Could you check a few things on this model? Use its own coordinates, in mm. Face numbers are marked on the shaded views. A direction names the side the tool comes from. Round coordinates to 2 decimals unless told otherwise and drop trailing zeros. Loops run counter-clockwise (first coordinate to the right, second up) from the corner with the lowest first, then second, coordinate; pieces in that order, holes last. Notation, with made-up numbers: (-21.75, -31.5) -> (31.25, -31.5) arc R10 cw to (31.25, -25.5) -> close; hole circle Ø11 at (-6.5, 23). An arc over 180 degrees is marked (long way). Write each question's results on one line, items separated by ' | '. Start each with the question number.
1) For P1, Ø4, axis at x = -231.5, y = 231.5, coming from the +Z side; P2, Ø8, axis at x = 100.5, z = -116.5, coming from the +Y side; P3, Ø5, axis at x = 156, y = 289.5, coming from the +Z side, each with a flat end and sliding along its axis, tell me the tip position at first contact or that it passes through.
2) Imagine slicing it at A-A, the plane y = 55.5. List the corners of the cut face in (x, z) for me.
3) We'd pull the mould along Z, two halves only. Please class the marked faces 1, 2 and 3: pulls with the +Z half, pulls with the -Z half, needs draft (parallel to the pull), parting line crosses it, or undercut.
4) Which directions (+Z, -Z, +X, -X, +Y, -Y) give clear straight access to the entire face, cutting with the end or side of a thin tool? Please do the marked faces 4 and 5.
5) Imagine slicing it at C-C, the plane z = -59.5. List the corners of the cut face in (x, y) for me.
6) If I drill on probe 1 along Z at (x, y) = (328, 100); probe 2 along Y at (x, z) = (423, 38); probe 3 along Z at (x, y) = (368, 274), over which ranges is the centre line in solid material (lowest first)?
7) Imagine slicing it at B-B, the plane x = -215.5. List the corners of the cut face in (y, z) for me, plus the area to 3 significant figures.
8) Imagine slicing it at D-D, the plane y = 220. List the corners of the cut face in (x, z) for me, plus the area to 3 significant figures.
Autodesk Inventor part; units mm, degrees
ref_plane "YZ Plane" through (0, 0, 0) normal (1, 0, 0) x (0, 1, 0)
ref_plane "XZ Plane" through (0, 0, 0) normal (0, 1, 0) x (-1, 0, 0)
ref_plane "XY Plane" through (0, 0, 0) normal (0, 0, 1) x (1, 0, 0)
sketch "Sketch1" plane through (0, 0, 0) normal (0, 1, 0) x (-1, 0, 0)
  line L0 (500, 200) -> (-500, 200)
  line L1 (-500, 200) -> (-500, -200)
  line L2 (-500, -200) -> (500, -200)
  line L3 (500, -200) -> (500, 200)
  line L4 (500, 200) -> (-500, -200) construction
  line L5 (-500, 200) -> (500, -200) construction
  point P0 (0, 0)
  dimension "d0" = 1000
  dimension "d1" = 400
extrude "Extrusion1" add sketch "Sketch1" along normal blind 300
fillet "Fillet1" radius 100 2 edges at (0, 300, 200) (0, 300, -200)
shell "Shell1" thickness 5 removed faces 3 at (-500, 100, -33.3333) at (166.6667, 0, 66.6667) at (500, 100, 33.3333)
sketch "Sketch2" plane through (0, 300, 0) normal (0, 1, 0) x (1, 0, 0)
  line L0 (-100, -50) -> (80, -50)
  line L1 (80, -50) -> (80, 50)
  line L2 (80, 50) -> (-100, 50)
  line L3 (-100, 50) -> (-100, -50)
  line L4 (-500, 100) -> (-500, -100)
  line L5 (500, -100) -> (-500, -100)
  point P0 (0, 0)
  dimension "d6" = 180
  dimension "d7" = 100
  dimension "d8" = 400
  dimension "d9" = 50
extrude "Extrusion2" add sketch "Sketch2" along normal blind 40
shell "Shell2" thickness 5 removed faces 1 at (-40, 340, 16.6667)
properties part number "GEAR PANEL"
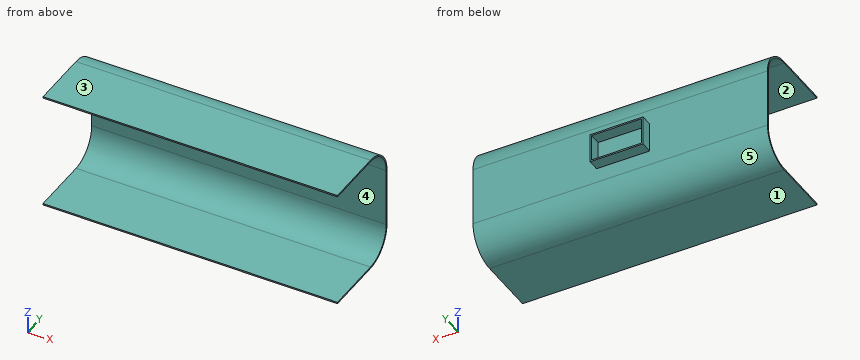
Checked values:
1) P1: z = 195.55 | P2: y = 299.22 | P3: z = 149.31
2) outline: (-500, -200) -> (500, -200) -> (500, -195) -> (-500, -195) -> close; (-500, 195) -> (500, 195) -> (500, 200) -> (-500, 200) -> close
3) face 1: pulls with the -Z half | face 2: undercut | face 3: pulls with the +Z half
4) face 4: +X, -X, -Y | face 5: -Z, +X, -X, +Y
5) outline: (-500, 295) -> (500, 295) -> (500, 300) -> (-500, 300) -> close
6) probe 1: -200 to -195, 195 to 200 | probe 2: 295 to 300 | probe 3: -167.26 to -159.57, 159.57 to 167.26
7) outline: (0, -200) -> (200, -200) arc R100 ccw to (300, -100) -> (300, 100) arc R100 ccw to (200, 200) -> (0, 200) -> (0, 195) -> (200, 195) arc R95 cw to (295, 100) -> (295, -100) arc R95 cw to (200, -195) -> (0, -195) -> close | area: 4,530 mm^2
8) outline: (-500, -197.98) -> (500, -197.98) -> (500, -192.87) -> (-500, -192.87) -> close; (-500, 192.87) -> (500, 192.87) -> (500, 197.98) -> (-500, 197.98) -> close | area: 10,200 mm^2
